```python
from build123d import *

# Parameters (mm, degrees)
CYLINDER_R     = 1.7
CYLINDER_DEPTH = 10


with BuildPart() as cilindro:
    # Cylinder → Cylinder (new body)
    with BuildSketch(Plane.XY.offset(-5)):
        Circle(CYLINDER_R)
    extrude(amount=CYLINDER_DEPTH)


with BuildPart() as cono:
    # Cone → Cone (revolve)
    with BuildSketch(Plane.XZ):
        Polygon((0, 0), (3, 0), (5, 3), (0, 3), align=None)
    revolve(axis=Axis((0, 0, 0), (0, 0, 1)))


with BuildPart() as tensioner:
    # Cone001 → Cone001 (revolve)
    with BuildSketch(Plane(origin=(0, 0, 0), x_dir=(1, 0, 0), z_dir=(0, 1, 0))):
        Polygon((0, 0), (3, 0), (5, 3), (0, 3), align=None)
    revolve(axis=Axis((0, 0, 0), (0, 0, -1)))

    # Fusion: union Cono
    add(cono.part)

    # Cut: cut Cilindro
    add(cilindro.part, mode=Mode.SUBTRACT)


solid = tensioner.part
```
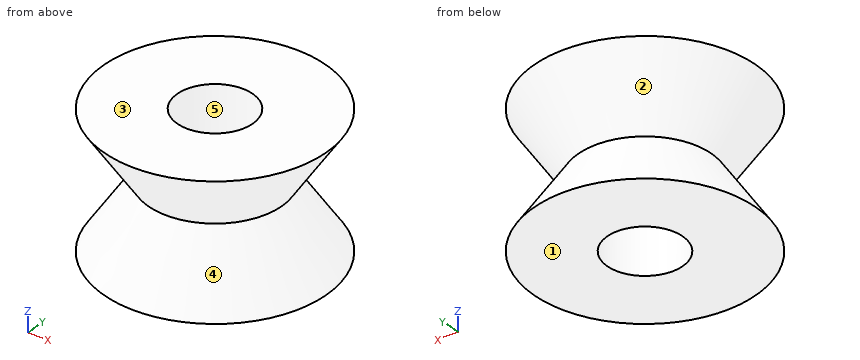
Work out the finished part from the listing and answer in its coordinate system (mm). Face numbers are marked on the shaded views. A direction names the side the tool comes from. Coordinates: 2 decimals unless noted, no trailing zeros. Loops run counter-clockwise (first coordinate to the right, second up) from the corner with the lowest first, then second, coordinate; pieces in that order, holes last.
1) Flat-ended cylindrical pins translate along their axes: pin 1 (2 mm diameter, centred on y = 1, z = -2, fed in from -X); pin 2 (2.5 mm diameter, centred on x = 0, y = 0, fed in from -Z); pin 3 (1 mm diameter, centred on y = -1, z = -2, fed in from -X). Find the tip coordinate at first contact, or state that the pin passes through.
Results:
pin 1: stops at x = -4.92
pin 2: passes through
pin 3: stops at x = -4.57
2) Section C-C (z = -1.2) is taken. Give the vertices of the cut face in (x, y), plus the area to 3 significant figures.
Results:
outline: circle Ø7.6 at (0, 0); hole circle Ø3.4 at (0, 0)
area: 36.3 mm2
3) For a pull along Y with two mould halves and no side action, classify the marked faces 3, 4 and 5 as +Y half, -Y half, draft (parallel to the pull), parting line (faces both ways), or undercut.
Results:
face 3: draft
face 4: parting line
face 5: undercut
4) Section D-D (z = 2.05) is taken. Give the vertices of the cut face in (x, y), plus the area to 3 significant figures.
Results:
outline: circle Ø8.73 at (0, 0); hole circle Ø3.4 at (0, 0)
area: 50.8 mm2
5) For the marked faces 1 and 2, determine the directions among +Z, -Z, +X, -X, +Y, -Y from which every point of the face is accessible in a straight line to the end or side of a thin tool.
Results:
face 1: -Z, +X, -X, +Y, -Y
face 2: none
6) Section A-A (x = 0) is taken. Give the vertices of the cut face in (y, z).
Results:
outline: (-5, -3) - (-1.7, -3) - (-1.7, 3) - (-5, 3) - (-3, 0) - close; (1.7, -3) - (5, -3) - (3, 0) - (5, 3) - (1.7, 3) - close
7) Consider probe 1 along Z at (x, y) = (2.75, -3.5); probe 2 along Y at (x, z) = (1.5, -2.7); probe 3 along Y at (x, z) = (0, -0.45). Determine where each line is inside the solid, lowest interval first.
Results:
probe 1: z = -3 to -2.18, 2.18 to 3
probe 2: y = -4.56 to -0.8, 0.8 to 4.56
probe 3: y = -3.3 to -1.7, 1.7 to 3.3
